from build123d import *

# Parameters (mm, degrees)
SKETCH1_R       = 3.5
SKETCH1_R_2     = 1.5
EXTRUDE_1_DEPTH = 3


with BuildPart() as part:
    # Sketch1 → Бобышка-Вытянуть1 (new body)
    with BuildSketch(Plane.XY):
        with BuildLine():
            Line((-24.498196466, 18.686253871), (-28.812938034, 21.763271713))
            ThreePointArc((-28.812938034, 21.763271713), (-34.033313652, 22.967935089), (-38.576502294, 20.128397731))
            Line((-38.576502294, 20.128397731), (-42.0602267, 15.24335277))
            ThreePointArc((-42.0602267, 15.24335277), (-43.264890076, 10.022977152), (-40.425352718, 5.47978851))
            Line((-40.425352718, 5.47978851), (-36.440527218, 2.638047245))
            ThreePointArc((-36.440527218, 2.638047245), (-34.281914219, 0.144259766), (-33.504872357, -3.061171876))
            Line((-33.504872357, -3.061171876), (-33.504872357, -48.061171876))
            ThreePointArc((-33.504872357, -48.061171876), (-34.969338451, -51.596705782), (-38.504872357, -53.061171876))
            Line((-38.504872357, -53.061171876), (-42.504872357, -53.061171876))
            ThreePointArc((-42.504872357, -53.061171876), (-47.454619825, -55.111424407), (-49.504872357, -60.061171876))
            Line((-49.504872357, -60.061171876), (-49.500334917, -60.235639257))
            Line((-49.500334917, -60.235639257), (-49.500334917, -66.108369799))
            Line((-49.500334917, -66.108369799), (-49.504872357, -66.28283718))
            ThreePointArc((-49.504872357, -66.28283718), (-47.454619825, -71.232584649), (-42.504872357, -73.28283718))
            Line((-42.504872357, -73.28283718), (-38.504872357, -73.28283718))
            ThreePointArc((-38.504872357, -73.28283718), (-34.969338451, -74.747303275), (-33.504872357, -78.28283718))
            Line((-33.504872357, -78.28283718), (-33.504872357, -123.28283718))
            ThreePointArc((-33.504872357, -123.28283718), (-34.281914219, -126.488268823), (-36.440527218, -128.982056301))
            Line((-36.440527218, -128.982056301), (-40.425352718, -131.823797566))
            ThreePointArc((-40.425352718, -131.823797566), (-43.264890076, -136.366986209), (-42.0602267, -141.587361827))
            Line((-42.0602267, -141.587361827), (-38.576502294, -146.472406787))
            ThreePointArc((-38.576502294, -146.472406787), (-34.033313652, -149.311944145), (-28.812938034, -148.107280769))
            Line((-28.812938034, -148.107280769), (-24.498196466, -145.030262927))
            ThreePointArc((-24.498196466, -145.030262927), (-21.740151192, -143.647892601), (-18.691989124, -143.172004528))
            Line((-18.691989124, -143.172004528), (46.687073776, -143.172004528))
            ThreePointArc((46.687073776, -143.172004528), (49.735235844, -143.647892601), (52.493281118, -145.030262927))
            Line((52.493281118, -145.030262927), (56.808022686, -148.107280769))
            ThreePointArc((56.808022686, -148.107280769), (62.028398304, -149.311944145), (66.571586947, -146.472406787))
            Line((66.571586947, -146.472406787), (70.055311352, -141.587361827))
            ThreePointArc((70.055311352, -141.587361827), (71.259974728, -136.366986209), (68.42043737, -131.823797566))
            Line((68.42043737, -131.823797566), (64.43561187, -128.982056301))
            ThreePointArc((64.43561187, -128.982056301), (62.276998871, -126.488268823), (61.499957009, -123.28283718))
            Line((61.499957009, -123.28283718), (61.499957009, -78.28283718))
            ThreePointArc((61.499957009, -78.28283718), (62.964423103, -74.747303275), (66.499957009, -73.28283718))
            Line((66.499957009, -73.28283718), (70.499957009, -73.28283718))
            ThreePointArc((70.499957009, -73.28283718), (75.449704478, -71.232584649), (77.499957009, -66.28283718))
            Line((77.499957009, -66.28283718), (77.495419569, -66.108369799))
            Line((77.495419569, -66.108369799), (77.495419569, -60.235639257))
            Line((77.495419569, -60.235639257), (77.499957009, -60.061171876))
            ThreePointArc((77.499957009, -60.061171876), (75.449704478, -55.111424407), (70.499957009, -53.061171876))
            Line((70.499957009, -53.061171876), (66.499957009, -53.061171876))
            ThreePointArc((66.499957009, -53.061171876), (62.964423103, -51.596705782), (61.499957009, -48.061171876))
            Line((61.499957009, -48.061171876), (61.499957009, -3.061171876))
            ThreePointArc((61.499957009, -3.061171876), (62.276998871, 0.144259766), (64.43561187, 2.638047245))
            Line((64.43561187, 2.638047245), (68.42043737, 5.47978851))
            ThreePointArc((68.42043737, 5.47978851), (71.259974728, 10.022977152), (70.055311352, 15.24335277))
            Line((70.055311352, 15.24335277), (66.571586947, 20.128397731))
            ThreePointArc((66.571586947, 20.128397731), (62.028398304, 22.967935089), (56.808022686, 21.763271713))
            Line((56.808022686, 21.763271713), (52.493281118, 18.686253871))
            ThreePointArc((52.493281118, 18.686253871), (49.735235844, 17.303883544), (46.687073776, 16.827995472))
            Line((46.687073776, 16.827995472), (-18.691989124, 16.827995472))
            ThreePointArc((-18.691989124, 16.827995472), (-21.740151192, 17.303883544), (-24.498196466, 18.686253871))
        make_face()
        with Locations((68.745419569, -63.172004528)):
            Circle(SKETCH1_R, mode=Mode.SUBTRACT)
        with Locations((-40.750334917, -63.172004528)):
            Circle(SKETCH1_R, mode=Mode.SUBTRACT)
        with Locations((33.997542326, 10.633411798)):
            Circle(SKETCH1_R_2, mode=Mode.SUBTRACT)
        with Locations((-6.002457674, 10.633411798)):
            Circle(SKETCH1_R_2, mode=Mode.SUBTRACT)
        with Locations((-33.194340596, 12.605443826)):
            Circle(SKETCH1_R, mode=Mode.SUBTRACT)
        with Locations(Location((61.189425248, 12.605443826, 0), (0, 0, 180))):
            Circle(SKETCH1_R, mode=Mode.SUBTRACT)
        with Locations(Location((-6.002457674, -136.977420854, 0), (0, 0, 180))):
            Circle(SKETCH1_R_2, mode=Mode.SUBTRACT)
        with Locations(Location((33.997542326, -136.977420854, 0), (0, 0, 180))):
            Circle(SKETCH1_R_2, mode=Mode.SUBTRACT)
        with Locations((-27.314872357, -100.78283718)):
            Circle(SKETCH1_R_2, mode=Mode.SUBTRACT)
        with Locations((55.309957009, -100.78283718)):
            Circle(SKETCH1_R_2, mode=Mode.SUBTRACT)
        with Locations((-27.314872357, -25.561171876)):
            Circle(SKETCH1_R_2, mode=Mode.SUBTRACT)
        with Locations((55.309957009, -25.561171876)):
            Circle(SKETCH1_R_2, mode=Mode.SUBTRACT)
        with Locations((-16.002457674, -118.172004528)):
            Circle(SKETCH1_R_2, mode=Mode.SUBTRACT)
        with Locations((36.997542326, -118.172004528)):
            Circle(SKETCH1_R_2, mode=Mode.SUBTRACT)
        with Locations((61.189425248, -138.949452883)):
            Circle(SKETCH1_R, mode=Mode.SUBTRACT)
        with Locations(Location((-33.194340596, -138.949452883, 0), (0, 0, 180))):
            Circle(SKETCH1_R, mode=Mode.SUBTRACT)
        with Locations((37.997542326, -18.172004528)):
            Circle(SKETCH1_R_2, mode=Mode.SUBTRACT)
        with Locations((-10.002457674, -18.172004528)):
            Circle(SKETCH1_R_2, mode=Mode.SUBTRACT)
        with Locations((32.99754233, -70.172004528)):
            Circle(SKETCH1_R_2, mode=Mode.SUBTRACT)
        with Locations((5.00245767, -70.172004528)):
            Circle(SKETCH1_R_2, mode=Mode.SUBTRACT)
        with BuildLine():
            Line((46.654347897, -45.877785269), (46.654347897, -57.916780859))
            ThreePointArc((46.654347897, -57.916780859), (45.604469083, -59.67668703), (43.557078164, -59.588904997))
            Line((43.557078164, -59.588904997), (26.221642115, -48.21316509))
            ThreePointArc((26.221642115, -48.21316509), (24.565051018, -46.408157708), (23.964816447, -44.032854745))
            Line((23.964816447, -44.032854745), (23.964816447, -36.732206564))
            Line((23.964816447, -36.732206564), (23.964816447, -30.674839138))
            ThreePointArc((23.964816447, -30.674839138), (25.060023185, -28.891205445), (27.1461656, -29.06101939))
            Line((27.1461656, -29.06101939), (44.60772078, -41.843235899))
            ThreePointArc((44.60772078, -41.843235899), (46.113432131, -43.615802114), (46.654347897, -45.877785269))
        make_face(mode=Mode.SUBTRACT)
        with BuildLine():
            Line((26.221642115, -98.352509271), (43.557078164, -86.976769364))
            ThreePointArc((43.557078164, -86.976769364), (45.604469083, -86.888987331), (46.654347897, -88.648893502))
            Line((46.654347897, -88.648893502), (46.654347897, -100.687889092))
            ThreePointArc((46.654347897, -100.687889092), (46.113432131, -102.949872247), (44.60772078, -104.722438462))
            Line((44.60772078, -104.722438462), (27.1461656, -117.50465497))
            ThreePointArc((27.1461656, -117.50465497), (25.060023185, -117.674468916), (23.964816447, -115.890835223))
            Line((23.964816447, -115.890835223), (23.964816447, -109.833467796))
            Line((23.964816447, -109.833467796), (23.964816447, -102.532819616))
            ThreePointArc((23.964816447, -102.532819616), (24.565051018, -100.157516653), (26.221642115, -98.352509271))
        make_face(mode=Mode.SUBTRACT)
        with BuildLine():
            Line((-18.659263245, -100.687889092), (-18.659263245, -88.648893502))
            ThreePointArc((-18.659263245, -88.648893502), (-17.60938443, -86.888987331), (-15.561993512, -86.976769364))
            Line((-15.561993512, -86.976769364), (1.773442538, -98.352509271))
            ThreePointArc((1.773442538, -98.352509271), (3.430033634, -100.157516653), (4.030268205, -102.532819616))
            Line((4.030268205, -102.532819616), (4.030268205, -109.833467796))
            Line((4.030268205, -109.833467796), (4.030268205, -115.890835223))
            ThreePointArc((4.030268205, -115.890835223), (2.935061467, -117.674468916), (0.848919052, -117.50465497))
            Line((0.848919052, -117.50465497), (-16.612636128, -104.722438462))
            ThreePointArc((-16.612636128, -104.722438462), (-18.118347479, -102.949872247), (-18.659263245, -100.687889092))
        make_face(mode=Mode.SUBTRACT)
        with BuildLine():
            Line((1.773442538, -48.21316509), (-15.561993512, -59.588904997))
            ThreePointArc((-15.561993512, -59.588904997), (-17.60938443, -59.67668703), (-18.659263245, -57.916780859))
            Line((-18.659263245, -57.916780859), (-18.659263245, -45.877785269))
            ThreePointArc((-18.659263245, -45.877785269), (-18.118347479, -43.615802114), (-16.612636128, -41.843235899))
            Line((-16.612636128, -41.843235899), (0.848919052, -29.06101939))
            ThreePointArc((0.848919052, -29.06101939), (2.935061467, -28.891205445), (4.030268205, -30.674839138))
            Line((4.030268205, -30.674839138), (4.030268205, -36.732206564))
            Line((4.030268205, -36.732206564), (4.030268205, -44.032854745))
            ThreePointArc((4.030268205, -44.032854745), (3.430033634, -46.408157708), (1.773442538, -48.21316509))
        make_face(mode=Mode.SUBTRACT)
        with BuildLine():
            Line((0.997542326, -10.561171876), (26.997542326, -10.561171876))
            ThreePointArc((26.997542326, -10.561171876), (28.411755888, -9.975385438), (28.997542326, -8.561171876))
            Line((28.997542326, -8.561171876), (28.997542326, -0.561171876))
            ThreePointArc((28.997542326, -0.561171876), (27.533076232, 2.97436203), (23.997542326, 4.438828124))
            Line((23.997542326, 4.438828124), (3.997542326, 4.438828124))
            ThreePointArc((3.997542326, 4.438828124), (0.46200842, 2.97436203), (-1.002457674, -0.561171876))
            Line((-1.002457674, -0.561171876), (-1.002457674, -8.561171876))
            ThreePointArc((-1.002457674, -8.561171876), (-0.416671236, -9.975385438), (0.997542326, -10.561171876))
        make_face(mode=Mode.SUBTRACT)
    extrude(amount=-EXTRUDE_1_DEPTH)


solid = part.part
Geometry check sheet. Reference: the model listing, model coordinates, mm. A direction names the side the tool comes from. Give positions to 0.01 mm unless a question says otherwise; leave off trailing zeros. Write each loop counter-clockwise with the first axis right and the second up, starting at its lowest first coordinate (ties: lowest second). Pieces come first, ordered by that corner, then holes. Notation, with made-up numbers: (43, 20.25) - (97, 20.25) arc R8 cw to (97, 33.25) - close; hole circle Ø11 at (0, 27.25). An arc over 180 degrees is marked (long way). Put each result on its own line as item: value.
1. Go/stop test with flat-tipped pins: pin 1 (1.5 mm diameter, centred on y = -107, z = -2, fed in from -X); pin 2 (0.9 mm diameter, centred on x = -40, z = -2, fed in from +Y); pin 3 (2.5 mm diameter, centred on x = -16, y = -118.17, fed in from -Z); pin 4 (0.9 mm diameter, centred on x = 28.5, z = -1, fed in from +Y). Record where each tip stops, or that it passes through.
Ans:
pin 1: stops at x = -33.5
pin 2: stops at y = 18.76
pin 3: passes through
pin 4: stops at y = 16.83
2. Thickness scan on line 1 (Y direction, x = 19, z = -1.4); line 2 (X direction, y = -30, z = -1.5); line 3 (X direction, y = -44.5, z = -2). Record the ranges inside material, lowest first.
Ans:
line 1: y = -143.17 to -10.56, 4.44 to 16.83
line 2: x = -33.5 to -0.43, 3.91 to 24.08, 28.43 to 61.5
line 3: x = -33.5 to -18.47, 4.01 to 23.99, 46.46 to 61.5
3. Sectioned sample at A-A, the plane x = 13. Enter the section's corners in (y, z).
Ans:
outline: (-143.17, -3) - (-10.56, -3) - (-10.56, 0) - (-143.17, 0) - close; (4.44, -3) - (16.83, -3) - (16.83, 0) - (4.44, 0) - close
4. Set-up check for faces 1 (the flat face through (-40.34, -144, -1.48)), 2 (the cylindrical face through (63.004, -51.635, -1.479)), 3 (the cylindrical face through (-34.931, -51.558, -1.479)), 4 (the flat face through (34.768, -92.744, -1.479)): record each of +Z, -Z, +X, -X, +Y, -Y from which the full face is reachable in a straight line by a thin tool's end or side.
Ans:
face 1: +Z, -Z, -X, -Y
face 2: +Z, -Z, +X
face 3: +Z, -Z, -X
face 4: +Z, -Z
5. Sectioned sample at D-D, the plane x = -22. Enter the section's corners in (y, z) (3 decimals).
Ans:
outline: (-143.735, -3) - (17.391, -3) - (17.391, 0) - (-143.735, 0) - close
6. Sectioned sample at C-C, the plane z = -1.2. Give the number of separate pieces and of enclosed holes in the cut face, plus the area to 3 significant figures.
Ans:
separate pieces: 1
enclosed holes: 25
area: 14,100 mm²
7. Sectioned sample at B-B, the plane y = -114. Enter the section's corners in (x, z), plus the area to 3 significant figures.
Ans:
outline: (-33.5, -3) - (-3.94, -3) - (-3.94, 0) - (-33.5, 0) - close; (4.03, -3) - (23.96, -3) - (23.96, 0) - (4.03, 0) - close; (31.93, -3) - (61.5, -3) - (61.5, 0) - (31.93, 0) - close
area: 237 mm²
